Part model, mm, in its own coordinate system. A direction names the side the tool comes from. Round coordinates to 2 decimals unless told otherwise and drop trailing zeros. Loops run counter-clockwise (first coordinate to the right, second up) from the corner with the lowest first, then second, coordinate; pieces in that order, holes last. Notation, with made-up numbers: (-38.5, 57.25) -> (-3.5, 57.25) arc R10 cw to (-3.5, 67.25) -> close; hole circle Ø3 at (29.5, 11). An arc over 180 degrees is marked (long way). Use a Markdown table: item, result. Add a question column.
Item 1: Flat gauge pins, fed straight in: pin 1 (1 mm diameter, centred on y = 82.5, z = -10, fed in from -X); pin 2 (2 mm diameter, centred on x = 41, z = -29, fed in from +Y); pin 3 (4 mm diameter, centred on x = 13, z = -11, fed in from +Y). Where does each tip first touch, or does it go through?
Item 2: Probe line 1 (X direction, y = 83, z = 0); line 2 (X direction, y = 139, z = -15). List the from-to ranges inside material, lowest first. Write a range as [from, to].
Item 3: Cut at C-C, the plane z = -10. List the corners of the cut face in (x, y) (1 decimal), plus the area to 3 significant figures.
Item 4: Two-plate mould, pull along X, no slides. Class faces 3 (the face through (42.36, 141.8, -7.81)), 4 (the face through (27.537, 184.246, -19.37)), 5 (the face through (-9, 0, -19)), 6 (the face through (-17.235, 5.916, -41.569)): pulls with the +X half, pulls with the -X half, needs draft (parallel to the pull), parting line crosses it, or undercut.
Item 5: Which spindle directions (+Z, -Z, +X, -X, +Y, -Y) get a long thin tool onto all of the face, cutting with end or side? Do faces 1 (the face through (-19, 12, -19)), 2 (the face through (-4.336, 60.84, 19.524)). Say none if no direction does.
Item 6: Cut at D-D, the plane z = 39. List the corners of the cut face in (x, y), plus the area to 3 significant figures.
Item 7: Cut at A-A, the plane z = 0. List the corners of the cut face in (x, y), plus the area to 3 significant figures.
Item 8: Cut at B-B, the plane y = 62. List the corners of the cut face in (x, z).
```python
from build123d import *

# Parameters (mm, degrees)
SKIZZE2_R                       = 26
SKIZZE2_R_2                     = 20
SKIZZE3_R                       = 45
SKIZZE3_R_2                     = 26
AUFSATZ_LINEAR_AUSTRAGEN1_DEPTH = 12
SKIZZE4_R                       = 45
SKIZZE4_R_2                     = 20
AUFSATZ_LINEAR_AUSTRAGEN2_DEPTH = 12


with BuildPart() as part:
    # Austragung-Dünn1: sweep along a path in Skizze1
    with BuildLine(Plane.XY) as austragung_d_nn1_path:
        Line((0, 0), (0, 120))
        ThreePointArc((0, 120), (6.02885683, 142.5), (22.5, 158.97114317))
        Line((22.5, 158.97114317), (47.61473671, 173.47114317))
    # Skizze2 → Austragung-Dünn1 (sweep)
    with BuildSketch(Plane(origin=(0, 0, 0), x_dir=(1, 0, 0), z_dir=(0, 1, 0))):
        Circle(SKIZZE2_R)
        Circle(SKIZZE2_R_2, mode=Mode.SUBTRACT)
    sweep(path=austragung_d_nn1_path.line)

    # Skizze3 → Aufsatz-Linear austragen1 (add)
    with BuildSketch(Plane.XZ):
        with Locations(Location((0, 0, 0), (0, 0, 270))):  # turned: the seam where the file's is
            Circle(SKIZZE3_R)
        with Locations(Location((0, 0, 0), (0, 0, 270))):  # turned: the seam where the file's is
            Circle(SKIZZE3_R_2, mode=Mode.SUBTRACT)
    extrude(amount=-AUFSATZ_LINEAR_AUSTRAGEN1_DEPTH)

    # Skizze4 → Aufsatz-Linear austragen2 (add)
    with BuildSketch(Plane(origin=(110.826260937, 63.985571585, 0), x_dir=(0, 0, -1), z_dir=(0.866025404, 0.5, 0))):
        with Locations(Location((0, 126.423048454, 0), (0, 0, 90))):  # turned: the seam where the file's is
            Circle(SKIZZE4_R)
        with Locations(Location((0, 126.423048454, 0), (0, 0, 90))):  # turned: the seam where the file's is
            Circle(SKIZZE4_R_2, mode=Mode.SUBTRACT)
    extrude(amount=-AUFSATZ_LINEAR_AUSTRAGEN2_DEPTH)


solid = part.part
```
A:
| question | item | result |
|---|---|---|
| 1 | pin 1 | stops at x = -24.2 |
| 1 | pin 2 | stops at y = 186.66 |
| 1 | pin 3 | stops at y = 182.22 |
| 2 | line 1 | x = [-26, -20], [20, 26] |
| 2 | line 2 | x = [-18.45, -10.04], [19.54, 30.73], [53.66, 67.52] |
| 3 | outline | (-43.9, 0) -> (-17.3, 0) -> (-17.3, 120) arc R62.3 cw to (13.8, 174) -> (39, 188.5) -> (25.7, 211.5) -> (15.3, 205.5) -> (25.2, 188.3) -> (10.5, 179.8) arc R69 ccw to (-24, 120) -> (-24, 12) -> (-43.9, 12) -> close; (17.3, 0) -> (43.9, 0) -> (43.9, 12) -> (24, 12) -> (24, 120) arc R21 cw to (34.5, 138.2) -> (49.2, 146.7) -> (59.2, 129.5) -> (69.6, 135.5) -> (56.3, 158.5) -> (31.2, 144) arc R27.7 ccw to (17.3, 120) -> close |
| 3 | area | 3,570 mm^2 |
| 4 | face 3 | undercut |
| 4 | face 4 | undercut |
| 4 | face 5 | needs draft |
| 4 | face 6 | parting line crosses it |
| 5 | face 1 | none |
| 5 | face 2 | -Y |
| 6 | outline | (-22.45, 0) -> (22.45, 0) -> (22.45, 12) -> (-22.45, 12) -> close; (26, 186.91) -> (48.45, 148.03) -> (58.84, 154.03) -> (36.39, 192.91) -> close |
| 6 | area | 1,080 mm^2 |
| 7 | outline | (-45, 0) -> (-20, 0) -> (-20, 120) arc R65 cw to (12.5, 176.29) -> (37.61, 190.79) -> (25.11, 212.44) -> (14.72, 206.44) -> (24.22, 189.99) -> (9.5, 181.49) arc R71 ccw to (-26, 120) -> (-26, 12) -> (-45, 12) -> close; (20, 0) -> (45, 0) -> (45, 12) -> (26, 12) -> (26, 120) arc R19 cw to (35.5, 136.45) -> (50.22, 144.95) -> (59.72, 128.5) -> (70.11, 134.5) -> (57.61, 156.15) -> (32.5, 141.65) arc R25 ccw to (20, 120) -> close |
| 7 | area | 3,270 mm^2 |
| 8 | outline | circle Ø52 at (0, 0); hole circle Ø40 at (0, 0) |
